Input: part model. Units: mm. Frame: model coordinates. A direction names the side the tool comes from. Round coordinates to 2 decimals unless told otherwise and drop trailing zeros. Write each loop counter-clockwise with the first axis right and the second up, starting at its lowest first coordinate (ties: lowest second). Pieces come first, ordered by that corner, then holes. Notation, with made-up numbers: (87, 12) -> (139, 12) arc R18 ccw to (139, 20) -> close; hole circle Ø9 at (-35, -26.75). An arc over 180 degrees is marked (long way). Write item = value, one per line.
```python
from build123d import *

# Parameters (mm, degrees)
SKETCH_1_W          = 520
SKETCH_1_H          = 150
EXTRUDE_1_DEPTH     = 80
SKETCH_3_W          = 520
SKETCH_3_H          = 150
EXTRUDE_2_DEPTH     = 40
CUT_EXTRUDE_1_DEPTH = 539.910938839
SKETCH_5_W          = 480
SKETCH_5_H          = 110
CUT_EXTRUDE_2_DEPTH = 70
SKETCH_7_W          = 480
SKETCH_7_H          = 55.028629816
CUT_EXTRUDE_3_DEPTH = 70
SKETCH_8_W          = 480
SKETCH_8_H          = 42.734816303
CUT_EXTRUDE_5_DEPTH = 30
SKETCH_9_W          = 480
SKETCH_9_H          = 45.831744101
CUT_EXTRUDE_6_DEPTH = 20
SKETCH_10_W         = 25
SKETCH_10_H         = 20
EXTRUDE_3_DEPTH     = 20
SKETCH_11_W         = 25
SKETCH_11_H         = 20
EXTRUDE_4_DEPTH     = 20


with BuildPart() as part:
    # 草圖1 → 填料-伸長1 (new body)
    with BuildSketch(Plane(origin=(0, 0, 0), x_dir=(1, 0, 0), z_dir=(0, 1, 0))):
        Rectangle(SKETCH_1_W, SKETCH_1_H)
    extrude(amount=EXTRUDE_1_DEPTH)

    # 草圖3 → 填料-伸長2 (add)
    with BuildSketch(Plane(origin=(0, 80, 0), x_dir=(1, 0, 0), z_dir=(0, 1, 0))):
        Rectangle(SKETCH_3_W, SKETCH_3_H)
    extrude(amount=EXTRUDE_2_DEPTH)

    # 草圖4 → 除料-伸長1 (cut, through all)
    with BuildSketch(Plane(origin=(260, 0, 0), x_dir=(0, 0, -1), z_dir=(1, 0, 0))):
        Polygon((-75, 80.706622888), (11.524395402, 120), (-75, 120), align=None)
    extrude(amount=-CUT_EXTRUDE_1_DEPTH, mode=Mode.SUBTRACT)

    # 草圖5 → 除料-伸長2 (cut)
    with BuildSketch(Plane(origin=(0, 0, 0), x_dir=(-1, 0, 0), z_dir=(0, -1, 0))):
        Rectangle(SKETCH_5_W, SKETCH_5_H)
    extrude(amount=-CUT_EXTRUDE_2_DEPTH, mode=Mode.SUBTRACT)

    # 草圖7 → 除料-伸長3 (cut)
    with BuildSketch(Plane(origin=(0, 95.144358744, 43.207966387), x_dir=(1, 0, 0), z_dir=(0, 0.9105087126935232, 0.4134898839260561))):
        with Locations((0, 12.597533586)):
            Rectangle(SKETCH_7_W, SKETCH_7_H)
    extrude(amount=-CUT_EXTRUDE_3_DEPTH, mode=Mode.SUBTRACT)

    # 草圖8 → 除料-伸長5 (cut)
    with BuildSketch(Plane.XZ.offset(-70)):
        with Locations((0, -33.632591848)):
            Rectangle(SKETCH_8_W, SKETCH_8_H)
    extrude(amount=-CUT_EXTRUDE_5_DEPTH, mode=Mode.SUBTRACT)

    # 草圖9 → 除料-伸長6 (cut)
    with BuildSketch(Plane(origin=(0, 16.585843578, -36.522187536), x_dir=(1, 0, 0), z_dir=(0, -0.4134898839260561, 0.9105087126935232))):
        with Locations((0, 81.579952556)):
            Rectangle(SKETCH_9_W, SKETCH_9_H)
    extrude(amount=-CUT_EXTRUDE_6_DEPTH, mode=Mode.SUBTRACT)

    # 草圖10 → 填料-伸長3 (add)
    with BuildSketch(Plane(origin=(0, 0, -85), x_dir=(-1, 0, 0), z_dir=(0, 0, -1))):
        with Locations((-187.5, 10)):
            Rectangle(SKETCH_10_W, SKETCH_10_H)
    extrude(amount=-EXTRUDE_3_DEPTH)

    # 草圖11 → 填料-伸長4 (add)
    with BuildSketch(Plane(origin=(0, 0, -85), x_dir=(-1, 0, 0), z_dir=(0, 0, -1))):
        with Locations((187.5, 10)):
            Rectangle(SKETCH_11_W, SKETCH_11_H)
    extrude(amount=-EXTRUDE_4_DEPTH)


solid = part.part
```
1) Draft query along Z for faces 1 (the face through (-4, 40, 75)), 2 (the face through (3, 35, 55)), 3 (the face through (1, 0, -59)), 4 (the face through (240, 57, 4)). Return one class per face: +Z half, -Z half, draft (parallel to the pull), parting line (faces both ways), or undercut.
Solutions:
face_1 = +Z half
face_2 = undercut
face_3 = draft
face_4 = undercut
2) First-contact query: P1, Ø3.5, axis at x = -116, z = 52.5, coming from the -Y side; P2, Ø1.5, axis at x = -58, z = -13.5, coming from the -Y side; P3, Ø3, axis at y = 8, z = -82, coming from the -X side. Flat tips, straight axial feed; report the tip coordinate or a pass-through.
Solutions:
P1 = 70
P2 = 114
P3 = -200
3) Cut plane A-A (x = -182). Return the cut outline in (y, z).
Solutions:
outline = (0, -85) -> (20, -85) -> (20, -75) -> (120, -75) -> (120, -11.52) -> (100, -20.61) -> (100, -55) -> (0, -55) -> close; (0, 55) -> (70, 55) -> (70, 48.17) -> (88.98, 56.79) -> (80.71, 75) -> (0, 75) -> close
4) Cut plane B-B (z = -3.5). Return the cut outline in (x, y).
Solutions:
outline = (-260, 0) -> (-240, 0) -> (-240, 116.36) -> (-260, 116.36) -> close; (240, 0) -> (260, 0) -> (260, 116.36) -> (240, 116.36) -> close
5) Access query for faces 5 (the face through (175, 10, -80)), 6 (the face through (-3.36, 79.62, 52.54)), 7 (the face through (-200, 10, -80)), 8 (the face through (200, 10, -80)). Directions: +Z, -Z, +X, -X, +Y, -Y. A direction counts if a zero-diameter tool reaches every point of the face in a straight line with its end or side. Return the directions, or none.
Solutions:
face_5 = -Z, +Y, -Y
face_6 = +Y
face_7 = -Z, -X, +Y, -Y
face_8 = -Z, +X, +Y, -Y
6) Line query: L1, parallel to X at y = 97, z = -2; L2, parallel to Z at x = 63.5, y = 16; L3, parallel to Y at x = 134, z = -43.5. Output: solid intervals per line, ascending. Write a range as from..to.
Solutions:
L1 = -260..-240, 240..260
L2 = -75..-55, 55..75
L3 = 100..120
7) Cut plane C-C (y = 37). Return the cut outline in (x, z), and give its area (3 significant figures).
Solutions:
outline = (-260, -75) -> (260, -75) -> (260, 75) -> (-260, 75) -> close; hole (-240, -55) -> (240, -55) -> (240, 55) -> (-240, 55) -> close
area = 25,200 mm^2
8) Cut plane D-D (x = 36.5). Return the cut outline in (y, z), and give its area (3 significant figures).
Solutions:
outline = (0, -75) -> (120, -75) -> (120, -11.52) -> (100, -20.61) -> (100, -55) -> (0, -55) -> close; (0, 55) -> (70, 55) -> (70, 48.17) -> (88.98, 56.79) -> (80.71, 75) -> (0, 75) -> close
area = 4,930 mm^2
